Part model, mm, in its own coordinate system. Coordinates: 2 decimals unless noted, no trailing zeros. Write each loop counter-clockwise with the first axis right and the second up, starting at its lowest first coordinate (ties: lowest second). Pieces come first, ordered by that corner, then holes. Notation, with made-up numbers: (27.5, -34) - (67.5, -34) arc R27 ccw to (67.5, -15) - close; hole circle Ø4 at (78, -10). An arc over 180 degrees is marked (long way). Use one line per item in the form item = value. Start each with the question number.
from build123d import *

# Parameters (mm, degrees)
SKIZZE1_W                       = 100
SKIZZE1_H                       = 30
AUFSATZ_LINEAR_AUSTRAGEN1_DEPTH = 3
SKIZZE2_R                       = 1.55
BOHRUNGEN_DEPTH                 = 105.446158378
SCHNITT_LINEAR_AUSTRAGEN3_DEPTH = 3


with BuildPart() as part:
    # Skizze1 → Aufsatz-Linear austragen1 (new body)
    with BuildSketch(Plane(origin=(0, 0, 0), x_dir=(0, 0, -1), z_dir=(1, 0, 0))):
        with Locations((50, 15)):
            Rectangle(SKIZZE1_W, SKIZZE1_H)
    extrude(amount=AUFSATZ_LINEAR_AUSTRAGEN1_DEPTH)

    # Skizze2 → Bohrungen (cut, through all)
    with BuildSketch(Plane(origin=(3, 0, 0), x_dir=(0, 0, -1), z_dir=(1, 0, 0))):
        with Locations((10, 22)):
            Circle(SKIZZE2_R)
        with Locations((31, 7)):
            Circle(SKIZZE2_R)
        with Locations((55.59187467, 7)):
            Circle(SKIZZE2_R)
        with Locations((80.183749339, 7)):
            Circle(SKIZZE2_R)
    extrude(amount=-BOHRUNGEN_DEPTH, mode=Mode.SUBTRACT)

    # Skizze6 → Schnitt-Linear austragen3 (cut)
    with BuildSketch(Plane.ZY):
        with BuildLine():
            ThreePointArc((-15.3, 19.295836543), (-4.05, 22), (-15.3, 24.704163457))
            ThreePointArc((-15.3, 24.704163457), (-19.05, 22), (-15.3, 19.295836543))
        make_face()
    extrude(amount=-SCHNITT_LINEAR_AUSTRAGEN3_DEPTH, mode=Mode.SUBTRACT)


solid = part.part
Q1. Slice it at B-B (z = -31). List the corners of the cut face in (x, y).
Q2. Slice it at D-D (x = 1.1). List the corners of the cut face in (y, z).
Q3. Slice it at C-C (y = 21). List the corners of the cut face in (x, z), plus the area to 3 significant figures.
Q4. Mould opens along Z. For faces 1 (the cylindrical face through (1.521, 7.466, -32.478)), 2 (the flat face through (3, 15, -49)), 3 (the flat face through (1, 15, -100)), 4 (the cylindrical face through (1.48, 22.08, -19.05)) say: released by +Z, released by -Z, zero draft, split by the parting line, or undercut.
Q5. Pin check, flat tip, straight feed: P1, Ø9.5, axis at y = 22, z = -10, coming from the +X side. Stop position of the tip, or through.
Q6. Slice it at A-A (y = 7). List the corners of the cut face in (x, z), plus the area to 3 significant figures.
Q7. Drill centre lines: probe 1 along Z at (x, y) = (0.65, 21.75); probe 2 along Y at (x, z) = (1.25, -31); probe 3 along Y at (x, z) = (0.95, -79). Where is each one in solid material? Low to high.
Solution:
q1.outline = (0, 0) - (3, 0) - (3, 5.45) - (0, 5.45) - close; (0, 8.55) - (3, 8.55) - (3, 30) - (0, 30) - close
q2.outline = (0, -100) - (30, -100) - (30, 0) - (0, 0) - close; hole circle Ø3.1 at (7, -80.18); hole circle Ø3.1 at (7, -55.59); hole circle Ø3.1 at (7, -31); hole (19.3, -15.3) arc R2.85 ccw (long way) to (24.7, -15.3) arc R5.95 ccw (long way) to start
q3.outline = (0, -100) - (3, -100) - (3, -18.87) - (0, -18.87) - close; (0, -4.13) - (3, -4.13) - (3, 0) - (0, 0) - close
q3.area = 256 mm2
q4.face_1 = undercut
q4.face_2 = zero draft
q4.face_3 = released by -Z
q4.face_4 = undercut
q5.P1 = through
q6.outline = (0, -100) - (3, -100) - (3, -81.73) - (0, -81.73) - close; (0, -78.63) - (3, -78.63) - (3, -57.14) - (0, -57.14) - close; (0, -54.04) - (3, -54.04) - (3, -32.55) - (0, -32.55) - close; (0, -29.45) - (3, -29.45) - (3, 0) - (0, 0) - close
q6.area = 272 mm2
q7.probe_1 = -100 to -19.04, -4.06 to 0
q7.probe_2 = 0 to 5.45, 8.55 to 30
q7.probe_3 = 0 to 6, 8 to 30
